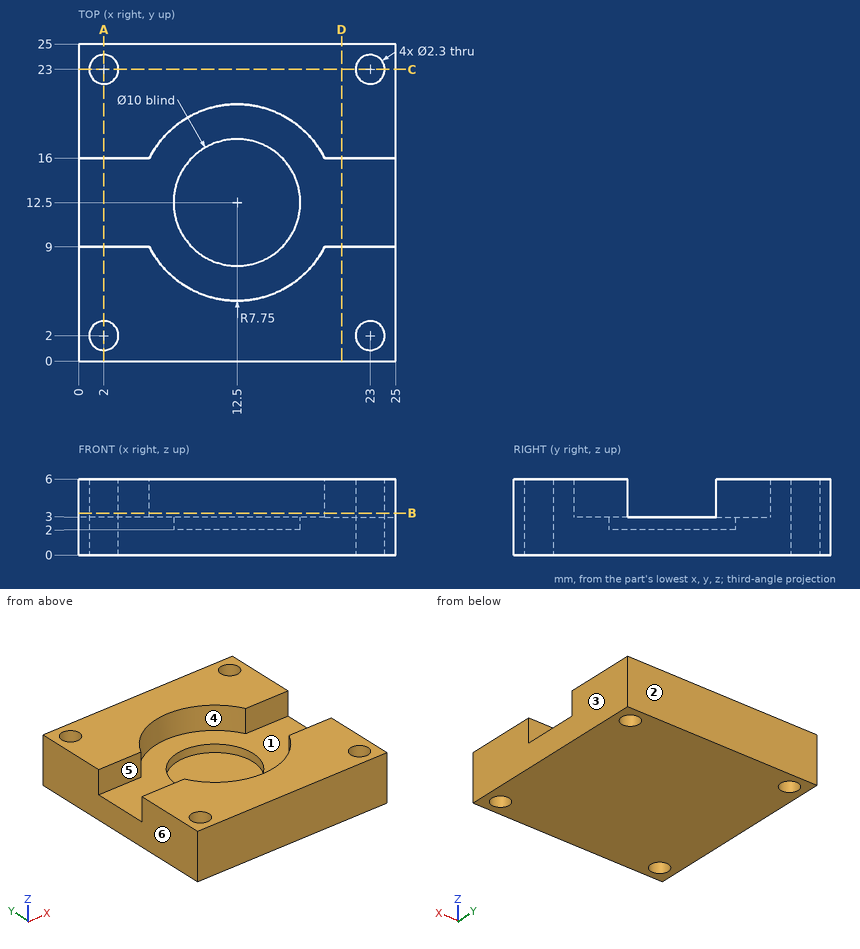
Print and shaded views of the part. All mm, measured from the part's lowest x, y and z. A direction names the side the tool comes from. Give positions to 0.01 mm unless a question says otherwise; leave off trailing zeros. Loops run counter-clockwise (first coordinate to the right, second up) from the corner with the lowest first, then second, coordinate; pieces in that order, holes last. Notation, with made-up numbers: (-38, 6) -> (-30, 6) arc R26 cw to (-30, 27) -> close; hole circle Ø2 at (-6.75, 84.25). An arc over 180 degrees is marked (long way). One line per question, with ' | ' between items. Start each with the question number.
1) Cut at B-B (z = 3.3). Give the cut face in (x, y), plus the area to 3 significant figures.
2) Pin check, flat tips, straight feed: pin 1 (2.5 mm diameter, centred on x = 23, y = 23, fed in from -Z); pin 2 (11 mm diameter, centred on x = 11.5, y = 12, fed in from +Z); pin 3 (2 mm diameter, centred on x = 2, y = 2, fed in from -Z). Stop position of each tip, or through.
3) Cut at A-A (x = 2). Give the cut face in (y, z), plus the area to 3 significant figures.
4) 3-axis set-ups, long thin cutter, end or side, ignore diameter. For the marked faces 4, 5 and 6: which of +Z, -Z, +X, -X, +Y, -Y reach the whole face in a straight line?
5) Cut at D-D (x = 20.75). Give the cut face in (y, z), plus the area to 3 significant figures.
6) Cut at C-C (y = 23). Give the cut face in (x, z).
7) Probe L1, parallel to Y at x = 2, z = 3.25; L2, parallel to Y at x = 2, z = 2.4; L3, parallel to Y at x = 12.5, z = 2.6. List the from-to ranges inside material, lowest first.
8) Two-plate mould, pull along X, no slides. Class the marked faces 1, 2 and 3: released by +X, released by -X, zero draft, split by the parting line, or undercut.
Return value:
1) outline: (0, 0) -> (25, 0) -> (25, 9) -> (19.41, 9) arc R7.75 cw to (5.59, 9) -> (0, 9) -> close; (0, 16) -> (5.59, 16) arc R7.75 cw to (19.41, 16) -> (25, 16) -> (25, 25) -> (0, 25) -> close; hole circle Ø2.3 at (2, 2); hole circle Ø2.3 at (2, 23); hole circle Ø2.3 at (23, 2); hole circle Ø2.3 at (23, 23) | area: 349 mm^2
2) pin 1: z = 0 | pin 2: z = 3 | pin 3: through
3) outline: (0, 0) -> (0.85, 0) -> (0.85, 6) -> (0, 6) -> close; (3.15, 0) -> (21.85, 0) -> (21.85, 6) -> (16, 6) -> (16, 3) -> (9, 3) -> (9, 6) -> (3.15, 6) -> close; (24.15, 0) -> (25, 0) -> (25, 6) -> (24.15, 6) -> close | area: 101 mm^2
4) face 4: +Z | face 5: +Z, +X, -X | face 6: +Z, -Z, -X, +Y, -Y
5) outline: (0, 0) -> (25, 0) -> (25, 6) -> (16, 6) -> (16, 3) -> (9, 3) -> (9, 6) -> (0, 6) -> close | area: 129 mm^2
6) outline: (0, 0) -> (0.85, 0) -> (0.85, 6) -> (0, 6) -> close; (3.15, 0) -> (21.85, 0) -> (21.85, 6) -> (3.15, 6) -> close; (24.15, 0) -> (25, 0) -> (25, 6) -> (24.15, 6) -> close
7) L1: 0 to 0.85, 3.15 to 9, 16 to 21.85, 24.15 to 25 | L2: 0 to 0.85, 3.15 to 21.85, 24.15 to 25 | L3: 0 to 7.5, 17.5 to 25
8) face 1: undercut | face 2: zero draft | face 3: released by +X
